Work out the finished part from the listing and answer in its coordinate system (mm). Face numbers are marked on the shaded views. A direction names the side the tool comes from. Give positions to 0.01 mm unless a question says otherwise; leave off trailing zeros. Write each loop counter-clockwise with the first axis right and the second up, starting at its lowest first coordinate (ties: lowest second). Pieces come first, ordered by that corner, then holes. Notation, with made-up numbers: (72, 49) -> (81, 49) arc R27 cw to (81, 67) -> close; hole circle Ø9 at (-6.75, 43.25). An arc over 180 degrees is marked (long way). Use a Markdown table: item, result. Add a question column.
Q1. Section D-D, the plane x = 50 is taken. Give the vertices of the cut face in (y, z), plus the area to 3 significant figures.
Q2. Section B-B, the plane y = -19 is taken. Give the vertices of the cut face in (x, z).
Q3. For a pull along Y with two mould halves and no side action, classify the marked faces 4, 5 and 6 as pulls with the +Y half, pulls with the -Y half, needs draft (parallel to the pull), parting line crosses it, or undercut.
Q4. Each of these flat-tipped pins is pushed along its axis until it touches: pin 1 Ø1.5 at (x, y) = (-28.5, 36) entering from +Z; pin 2 Ø20 at (x, z) = (-4.5, 13.5) entering from +Y; pin 3 Ø3 at (x, y) = (-30, 46.5) entering from +Z; pin 4 Ø1.5 at (y, z) = (-20, 7) entering from +X. Where does it stop, or does it pass through?
Q5. Section A-A, the plane x = 5 is taken. Give the vertices of the cut face in (y, z).
Q6. For the marked faces 1, 2 and 3, determine the directions among +Z, -Z, +X, -X, +Y, -Y from which every point of the face is accessible in a straight line to the end or side of a thin tool.
Q7. Consider line 1 (Z direction, x = 43.5, y = -3); line 2 (Y direction, x = -25, z = -30.5); line 3 (X direction, y = -15.5, z = 10.5). Determine where each line is inside the solid, lowest interval first.
Q8. Section C-C, the plane z = -10.5 is taken. Give the vertices of the cut face in (x, y), plus the area to 3 significant figures.
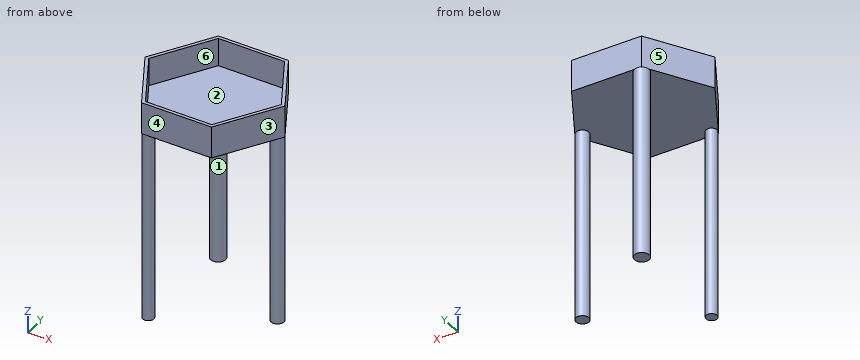
from build123d import *

# Parameters (mm, degrees)
F1_DEPTH = 25
F2_DEPTH = 3
F3_R     = 4.38636
F4_DEPTH = 150
F3_R_2   = 5.18705
F5_DEPTH = 150
F3_R_3   = 5.885261
F6_DEPTH = 150


with BuildPart() as f1:
    # F0 (on Top) → F1 (new body)
    with BuildSketch(Plane.XY):
        Polygon((28, -48.497423), (56, 0), (28, 48.497423), (-28, 48.497423), (-56, 0), (-28, -48.497423), align=None)
        Polygon((26.5, 45.899346), (53, 0), (26.5, -45.899346), (-26.5, -45.899346), (-53, 0), (-26.5, 45.899346), align=None, mode=Mode.SUBTRACT)
    extrude(amount=F1_DEPTH)

    # F0 (on Top) → F2 (join)
    with BuildSketch(Plane.XY):
        Polygon((26.5, -45.899346), (53, 0), (26.5, 45.899346), (-26.5, 45.899346), (-53, 0), (-26.5, -45.899346), align=None)
    extrude(amount=F2_DEPTH)

    # F3 (on Top) → F4 (join)
    with BuildSketch(Plane.XY):
        with Locations((-25.37145, -44.025768)):
            Circle(F3_R)
    extrude(amount=-F4_DEPTH)

    # F3 (on Top) → F5 (join)
    with BuildSketch(Plane.XY):
        with Locations((50, 0)):
            Circle(F3_R_2)
    extrude(amount=-F5_DEPTH)

    # F3 (on Top) → F6 (join)
    with BuildSketch(Plane.XY):
        with Locations((-25.37145, -44.025768)):
            Circle(F3_R)
        with Locations((50, 0)):
            Circle(F3_R_2)
        with Locations((-24.971633, 43.317751)):
            Circle(F3_R_3)
    extrude(amount=-F6_DEPTH)


solid = f1.part
Result set:
| question | item | result |
|---|---|---|
| 1 | outline | (-10.39, 0) -> (-5.19, 0) -> (-5.19, -150) -> (5.19, -150) -> (5.19, 0) -> (10.39, 0) -> (10.39, 25) -> (5.2, 25) -> (5.2, 3) -> (-5.2, 3) -> (-5.2, 25) -> (-10.39, 25) -> close |
| 1 | area | 1,850 mm2 |
| 2 | outline | (-45.03, 0) -> (45.03, 0) -> (45.03, 25) -> (42.03, 25) -> (42.03, 3) -> (-42.03, 3) -> (-42.03, 25) -> (-45.03, 25) -> close |
| 3 | face 4 | pulls with the -Y half |
| 3 | face 5 | pulls with the +Y half |
| 3 | face 6 | undercut |
| 4 | pin 1 | stops at z = 3 |
| 4 | pin 2 | stops at y = 48.5 |
| 4 | pin 3 | stops at z = 25 |
| 4 | pin 4 | stops at x = 44.89 |
| 5 | outline | (-48.5, 0) -> (48.5, 0) -> (48.5, 25) -> (45.9, 25) -> (45.9, 3) -> (-45.9, 3) -> (-45.9, 25) -> (-48.5, 25) -> close |
| 6 | face 1 | -Z |
| 6 | face 2 | +Z |
| 6 | face 3 | +Z, -Z, +X, -Y |
| 7 | line 1 | z = 0 to 3 |
| 7 | line 2 | y = -48.4 to -39.66, 37.43 to 49.2 |
| 7 | line 3 | x = -47.05 to -44.05, 44.05 to 47.05 |
| 8 | outline | circle Ø11.77 at (-24.97, 43.32); circle Ø8.77 at (-25.37, -44.03); circle Ø10.37 at (50, 0) |
| 8 | area | 254 mm2 |
